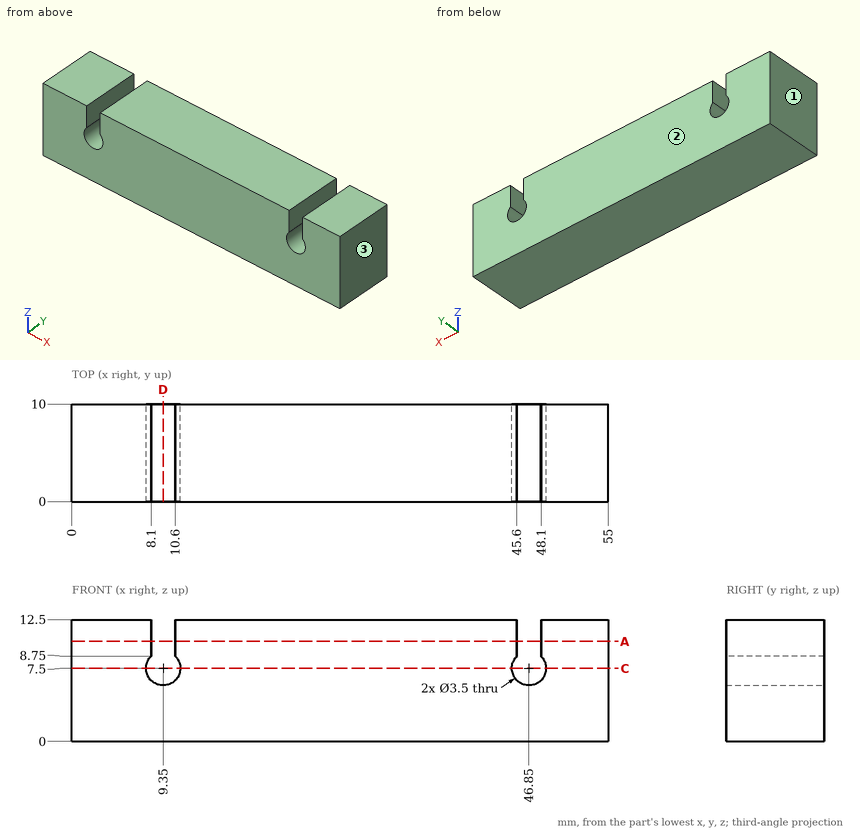
Could you check a few things on this drawing? It's one solid part, dimensions in mm from its lowest x, y, z. Coordinates: 2 decimals unless noted, no trailing zeros. Order: outer loops, then holes, each group sorted by start corner. A loop starts at its lowest first (then second) coordinate and runs counter-clockwise, first axis right, second up.
1) Imagine slicing it at A-A on z = 10.25. List the corners of the cut face in (x, y) for me.
2) We'd pull the mould along X, two halves only. Please class the marked faces 1, 2 and 3: +X half, -X half, draft (parallel to the pull), parting line (faces both ways), or undercut.
3) Will these pins go through, and if not, where does the flat tip stop? pin 1 (3 mm diameter, centred on x = 46.85, z = 7.5, fed in from -Y); pin 2 (2 mm diameter, centred on x = 47, y = 6.5, fed in from +Z).
4) Imagine slicing it at C-C on z = 7.5. List the corners of the cut face in (x, y) for me, and give its area (3 significant figures).
5) Imagine slicing it at D-D on x = 9.35. List the corners of the cut face in (y, z) for me.
6) I need wall thicknesses on line 1 (X direction, y = 4.5, z = 7.5); line 2 (X direction, y = 3.5, z = 11.75); line 3 (Z direction, x = 46.85, y = 3). Which ranges of each line are inside material? Lowest first, please.
Response values:
1. outline: (0, 0) - (8.1, 0) - (8.1, 10) - (0, 10) - close; (10.6, 0) - (45.6, 0) - (45.6, 10) - (10.6, 10) - close; (48.1, 0) - (55, 0) - (55, 10) - (48.1, 10) - close
2. face 1: -X half
2. face 2: draft
2. face 3: +X half
3. pin 1: passes through
3. pin 2: stops at z = 6.18
4. outline: (0, 0) - (7.6, 0) - (7.6, 10) - (0, 10) - close; (11.1, 0) - (45.1, 0) - (45.1, 10) - (11.1, 10) - close; (48.6, 0) - (55, 0) - (55, 10) - (48.6, 10) - close
4. area: 480 mm2
5. outline: (0, 0) - (10, 0) - (10, 5.75) - (0, 5.75) - close
6. line 1: x = 0 to 7.6, 11.1 to 45.1, 48.6 to 55
6. line 2: x = 0 to 8.1, 10.6 to 45.6, 48.1 to 55
6. line 3: z = 0 to 5.75
